```python
from build123d import *

# Parameters (mm, degrees)
ESQUISSE1_W        = 35
ESQUISSE1_H        = 10
ESQUISSE1_R        = 2.5
BOSS_EXTRU_1_DEPTH = 5
CONG_1_R           = 2
CONG_2_R           = 2
CONG_3_R           = 2
CONG_4_R           = 2


with BuildPart() as part:
    # Esquisse1 → Boss.-Extru.1 (new body)
    with BuildSketch(Plane.XY):
        with Locations((1.158413849, 3.369565217)):
            Rectangle(ESQUISSE1_W, ESQUISSE1_H)
        with Locations((-11.341586151, 3.369565217)):
            Circle(ESQUISSE1_R, mode=Mode.SUBTRACT)
        with Locations(Location((13.658413849, 3.369565217, 0), (0, 0, 180))):
            Circle(ESQUISSE1_R, mode=Mode.SUBTRACT)
    extrude(amount=BOSS_EXTRU_1_DEPTH)

    # Congé1
    cong_1_edges = [part.edges().sort_by_distance(p)[0] for p in [
        (-16.341586151, 8.369565217, 2.5),
    ]]
    fillet(cong_1_edges, radius=CONG_1_R)

    # Congé2
    cong_2_edges = [part.edges().sort_by_distance(p)[0] for p in [
        (-16.341586151, -1.630434783, 2.5),
    ]]
    fillet(cong_2_edges, radius=CONG_2_R)

    # Congé3
    cong_3_edges = [part.edges().sort_by_distance(p)[0] for p in [
        (18.658413849, 8.369565217, 2.5),
    ]]
    fillet(cong_3_edges, radius=CONG_3_R)

    # Congé4
    cong_4_edges = [part.edges().sort_by_distance(p)[0] for p in [
        (18.658413849, -1.630434783, 2.5),
    ]]
    fillet(cong_4_edges, radius=CONG_4_R)


solid = part.part
```
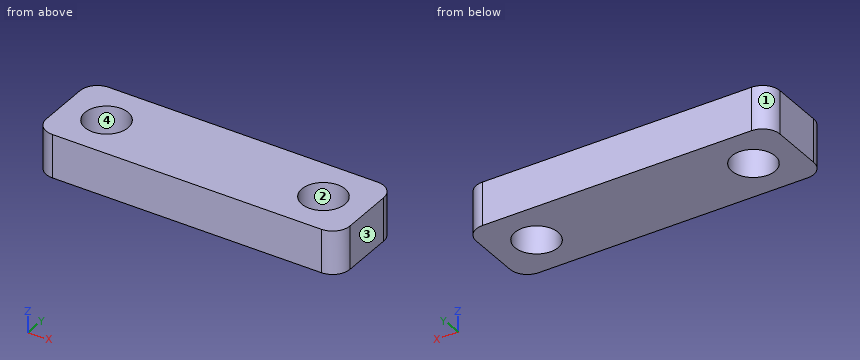
Check sheet for the modelled part. Datum: model origin and axes. Units: mm. Face numbers are marked on the shaded views. Coordinates: 2 decimals unless noted, no trailing zeros. Loops run counter-clockwise (first coordinate to the right, second up) from the corner with the lowest first, then second, coordinate; pieces in that order, holes last. Notation, with made-up numbers: M 85.25,73.5 L 128.25,73.5 A27 cw 128.25,107.5 Z; hole C -17,-4.75 d8. An arc over 180 degrees is marked long. Answer as a JSON object with one key per item and string values.
1. Sectioned sample at D-D on y = 3. Record the cut outline in (x, z), and give its area (3 significant figures).
Outcome:
{"outline": "M -16.34,0 L -13.81,0 L -13.81,5 L -16.34,5 Z; M -8.87,0 L 11.19,0 L 11.19,5 L -8.87,5 Z; M 16.13,0 L 18.66,0 L 18.66,5 L 16.13,5 Z", "area": "126 mm²"}
2. Sectioned sample at B-B on x = -12.5. Record the cut outline in (y, z).
Outcome:
{"outline": "M -1.63,0 L 1.15,0 L 1.15,5 L -1.63,5 Z; M 5.58,0 L 8.37,0 L 8.37,5 L 5.58,5 Z"}
3. Depth check by flat-ended pin: P1, Ø1, axis at x = -1, y = 1.5, coming from the -Z side. Enter the tip coordinate at first touch or a pass-through.
Outcome:
{"P1": "z = 0"}
4. Scan lines: L1, parallel to X at y = 2.5, z = 3.5; L2, parallel to X at y = 1.5, z = 4.6; L3, parallel to Y at x = 14, z = 0.55. Record each from-to range of solid material in increasing order. Write a range as from..to.
Outcome:
{"L1": "-16.34..-13.69, -9..11.31, 16..18.66", "L2": "-16.34..-13, -9.68..12, 15.32..18.66", "L3": "-1.63..0.89, 5.85..8.37"}
5. Sectioned sample at C-C on z = 2.95. Record the cut outline in (x, y), and give its area (3 significant figures).
Outcome:
{"outline": "M -16.34,0.37 A2 ccw -14.34,-1.63 L 16.66,-1.63 A2 ccw 18.66,0.37 L 18.66,6.37 A2 ccw 16.66,8.37 L -14.34,8.37 A2 ccw -16.34,6.37 Z; hole C -11.34,3.37 d5; hole C 13.66,3.37 d5", "area": "307 mm²"}
6. Release check for a two-part mould opening along X. For the marked faces 1, 2, 3 and 4 record: pulls with the +X half, pulls with the -X half, needs draft (parallel to the pull), parting line crosses it, or undercut.
Outcome:
{"face 1": "pulls with the -X half", "face 2": "undercut", "face 3": "pulls with the +X half", "face 4": "undercut"}
7. Sectioned sample at A-A on y = 5.5. Record the cut outline in (x, z).
Outcome:
{"outline": "M -16.34,0 L -12.65,0 L -12.65,5 L -16.34,5 Z; M -10.03,0 L 12.35,0 L 12.35,5 L -10.03,5 Z; M 14.97,0 L 18.66,0 L 18.66,5 L 14.97,5 Z"}
